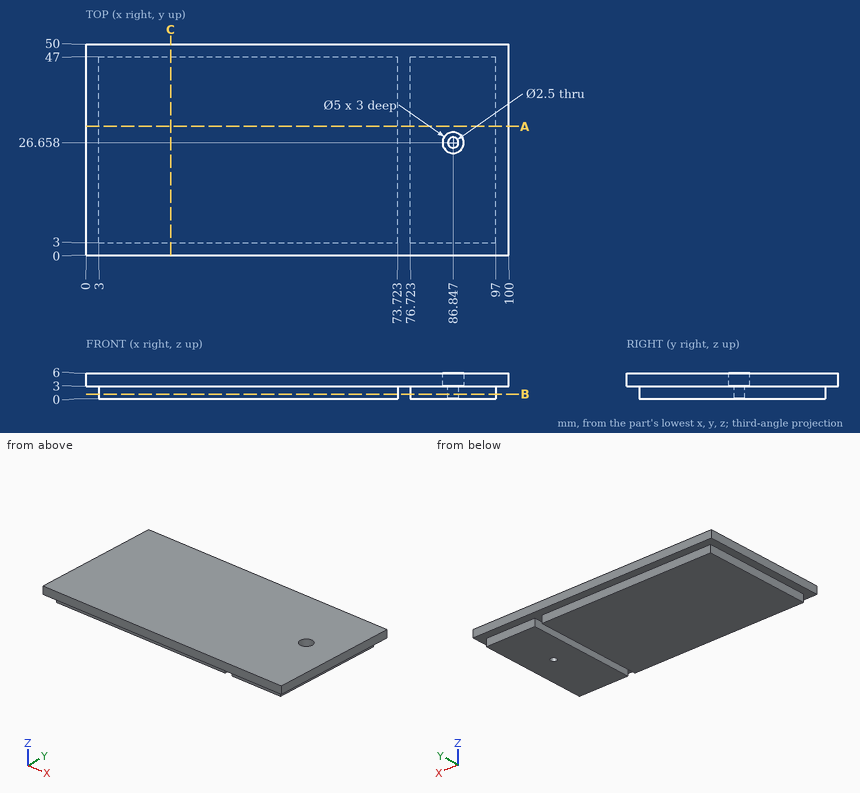
Part print with two shaded views. Sizes in mm from the minimum x, y, z corner. Coordinates: 2 decimals unless noted, no trailing zeros. Loops run counter-clockwise (first coordinate to the right, second up) from the corner with the lowest first, then second, coordinate; pieces in that order, holes last. Notation, with made-up numbers: M 13.25,-2.5 L 63.25,-2.5 A19 ccw 63.25,19.5 Z; hole C 80.25,65.25 d3. An arc over 180 degrees is marked long. Use CSV: the item, a comma, the result in double quotes. Start each with the question number.
1. Flat gauge pins, fed straight in: pin 1 (2 mm diameter, centred on x = 86.85, y = 26.66, fed in from -Z); pin 2 (2.5 mm diameter, centred on x = 89.5, z = 1.5, fed in from +Y); pin 3 (0.9 mm diameter, centred on y = 18.5, z = 1.5, fed in from -X); pin 4 (2.5 mm diameter, centred on y = 33.5, z = 1.5, fed in from +X). Where does each tip first touch, or does it go through?
2. Band-saw the part on C-C, the plane x = 20. List the corners of the cut face in (y, z).
3. Band-saw the part on A-A, the plane y = 30.5. List the corners of the cut face in (x, z).
4. Band-saw the part on B-B, the plane z = 1.1. List the corners of the cut face in (x, y).
5. Probe probe 1 along X at (y, z) = (42, 2.5); probe 2 along X at (y, z) = (26.5, 2.9); probe 3 along Y at (x, z) = (87, 3.55). List the from-to ranges inside material, lowest first. Write a range as [from, to].
Entries:
1,pin 1,"passes through"
1,pin 2,"stops at y = 47"
1,pin 3,"stops at x = 3"
1,pin 4,"stops at x = 97"
2,outline,"M 0,3 L 3,3 L 3,0 L 47,0 L 47,3 L 50,3 L 50,6 L 0,6 Z"
3,outline,"M 0,3 L 3,3 L 3,0 L 73.72,0 L 73.72,3 L 76.72,3 L 76.72,0 L 97,0 L 97,3 L 100,3 L 100,6 L 0,6 Z"
4,outline,"M 3,3 L 73.72,3 L 73.72,47 L 3,47 Z; M 76.72,3 L 97,3 L 97,47 L 76.72,47 Z; hole C 86.85,26.66 d2.5"
5,probe 1,"x = [3, 73.72], [76.72, 97]"
5,probe 2,"x = [3, 73.72], [76.72, 85.61], [88.09, 97]"
5,probe 3,"y = [0, 24.16], [29.15, 50]"
